from build123d import *

# Parameters (mm, degrees)
BOSS_EXTRUDE1_DEPTH     = 101
CUT_EXTRUDE1_START      = -32.5
SKETCH3_R               = 7.5
SKETCH3_R_2             = 5.975
CUT_EXTRUDE1_DEPTH      = 32.5
SKETCH4_R               = 7.5
SKETCH4_R_2             = 5.975
CUT_EXTRUDE2_DEPTH      = 32.5
CUT_EXTRUDE3_DEPTH      = 102.900993616
CUT_EXTRUDE3_DEPTH_BACK = 102.900993616
SKETCH5_W               = 8.2
SKETCH5_H               = 30.2
CUT_EXTRUDE4_DEPTH      = 103.382859894
CUT_EXTRUDE4_DEPTH_BACK = 103.382859894
HOLE1_D                 = 3.2
HOLE1_CSINK_D           = 6.3
HOLE1_CSINK_ANGLE       = 90


with BuildPart() as part:
    # Sketch1 → Boss-Extrude1 (new body)
    with BuildSketch(Plane.XY):
        with BuildLine():
            ThreePointArc((7.5, 0), (-1.941142838, 7.244443697), (-6.495190528, -3.75))
            Line((-6.495190528, -3.75), (6.495190528, -3.75))
            ThreePointArc((6.495190528, -3.75), (7.244443697, -1.941142838), (7.5, 0))
        make_face()
    extrude(amount=BOSS_EXTRUDE1_DEPTH)

    # Sketch3 → Cut-Extrude1 (cut)
    with BuildSketch(Plane.XY.offset(101).offset(CUT_EXTRUDE1_START)):
        Circle(SKETCH3_R)
        Circle(SKETCH3_R_2, mode=Mode.SUBTRACT)
    extrude(amount=CUT_EXTRUDE1_DEPTH, mode=Mode.SUBTRACT)

    # Sketch4 → Cut-Extrude2 (cut)
    with BuildSketch(Plane(origin=(0, 0, 0), x_dir=(-1, 0, 0), z_dir=(0, 0, -1))):
        Circle(SKETCH4_R)
        Circle(SKETCH4_R_2, mode=Mode.SUBTRACT)
    extrude(amount=-CUT_EXTRUDE2_DEPTH, mode=Mode.SUBTRACT)

    # Sketch5 → Cut-Extrude3 (cut, two sides: drawn at the far end of the back side and taken through both)
    with BuildSketch(Plane.XZ.offset(3.75).offset(-CUT_EXTRUDE3_DEPTH_BACK)):
        with Locations((0, 50.5)):
            Rectangle(SKETCH5_W, SKETCH5_H)
    extrude(amount=CUT_EXTRUDE3_DEPTH + CUT_EXTRUDE3_DEPTH_BACK, mode=Mode.SUBTRACT)

    # Sketch10 → Cut-Extrude4 (cut, two sides: drawn at the far end of the back side and taken through both)
    with BuildSketch(Plane.ZY.offset(7.5).offset(-CUT_EXTRUDE4_DEPTH_BACK)):
        with BuildLine():
            ThreePointArc((45.325, 2.112742786), (43.5, 3.937742786), (41.675, 2.112742786))
            Line((41.675, 2.112742786), (45.325, 2.112742786))
        make_face()
        with BuildLine():
            Line((45.325, 2.112742786), (41.675, 2.112742786))
            ThreePointArc((41.675, 2.112742786), (43.5, 0.287742786), (45.325, 2.112742786))
        make_face()
        with BuildLine():
            ThreePointArc((59.325, 2.112742786), (57.5, 3.937742786), (55.675, 2.112742786))
            Line((55.675, 2.112742786), (59.325, 2.112742786))
        make_face()
        with BuildLine():
            Line((59.325, 2.112742786), (55.675, 2.112742786))
            ThreePointArc((55.675, 2.112742786), (57.5, 0.287742786), (59.325, 2.112742786))
        make_face()
    extrude(amount=CUT_EXTRUDE4_DEPTH + CUT_EXTRUDE4_DEPTH_BACK, mode=Mode.SUBTRACT)

    # Hole1 (through all)
    with Locations(Plane(origin=(0, -3.75, 82.5), x_dir=(0, 0, -1), z_dir=(0, -1, 0))):
        with Locations((0, 0), (64, 0)):
            CounterSinkHole(HOLE1_D / 2, HOLE1_CSINK_D / 2, counter_sink_angle=HOLE1_CSINK_ANGLE)


solid = part.part
For this review, take the finished solid that the model builds, in its own axes (mm). A direction names the side the tool comes from. Round coordinates to 2 decimals unless told otherwise and drop trailing zeros. Loops run counter-clockwise (first coordinate to the right, second up) from the corner with the lowest first, then second, coordinate; pieces in that order, holes last. Notation, with made-up numbers: (0.5, 83.25) - (21.5, 83.25) arc R24 cw to (21.5, 99.25) - close; hole circle Ø10 at (-10, 63.25). An arc over 180 degrees is marked (long way). Put each result on its own line as item: value. Start each with the question number.
1. Consider section A-A on z = 82.5. State the section outline as (x, y) points (3 decimals).
2. For probe 1 along Z at (x, y) = (0, 3.5); probe 2 along X at (y, z) = (0.5, 35.5); probe 3 along Z at (x, y) = (-1.75, -1), list the stretches that pass through material, from the lowest coordinate up. Write a range as [from, to].
3. For faces 5 (the flat face through (4.1, 1, 50)), 6 (the cylindrical face through (5.8, 0.3, 57.7)), 7 (the cylindrical face through (-0.19, 5.97, 16.02)), list the 3-axis set-ups (+Z, -Z, +X, -X, +Y, -Y) from which the entire face can be reached by the end or side of a thin tool; tool diameter is ignored.
4. Consider section C-C on z = 57.5. State the section outline as (x, y) points.
5. Insertion check: P1, Ø1, axis at y = 5, z = 28, coming from the +X side; P2, Ø3.5, axis at x = 0, z = 82.5, coming from the +Y side (3 decimals); P3, Ø2, axis at y = 6.5, z = 61, coming from the -X side; P4, Ø3, axis at y = 2.11, z = 43.5, coming from the +X side. Each pin has a flat end and moves straight along its axis. Give the tip position at first contact, or say it passes through.
6. Consider section B-B on x = 0. State the section outline as (y, z) points (3 decimals).
7. Mouldability with a two-part tool opening along Z and no side actions: class faces 1 (the flat face through (0, 1, 101)), 2 (the flat face through (-4.4, -3.75, 49.8)), 3 (the cylindrical face through (5.8, 0.3, 43.7)), 4 (the flat face through (-4.1, 1, 50)) as +Z half, -Z half, draft (parallel to the pull), parting line (faces both ways), or undercut.
Result sheet:
1. outline: (-4.652, -3.75) - (-3.15, -3.75) - (-1.6, -2.2) - (-1.6, 5.757) arc R5.975 ccw to start; (1.6, -2.2) - (3.15, -3.75) - (4.652, -3.75) arc R5.975 ccw to (1.6, 5.757) - close
2. probe 1: [0, 16.9], [20.1, 35.4], [65.6, 80.9], [84.1, 101]
2. probe 2: [-7.48, -4.1], [4.1, 7.48]
2. probe 3: [0, 35.4], [65.6, 101]
3. face 5: +Y, -Y
3. face 6: +X, -X
3. face 7: -Z
4. outline: (-7.49, 0.29) arc R7.5 ccw to (-6.5, -3.75) - (-4.1, -3.75) - (-4.1, 0.29) - close; (-6.38, 3.94) - (-4.1, 3.94) - (-4.1, 6.28) arc R7.5 ccw to start; (4.1, -3.75) - (6.5, -3.75) arc R7.5 ccw to (7.49, 0.29) - (4.1, 0.29) - close; (4.1, 3.94) - (6.38, 3.94) arc R7.5 ccw to (4.1, 6.28) - close
5. P1: x = 3.93
5. P2: y = 5.975
5. P3: x = -5.1
5. P4: through
6. outline: (-3.75, 0) - (5.975, 0) - (5.975, 16.9) - (-2.2, 16.9) - (-3.75, 15.35) - close; (-3.75, 21.65) - (-2.2, 20.1) - (5.975, 20.1) - (5.975, 32.5) - (7.5, 32.5) - (7.5, 35.4) - (-3.75, 35.4) - close; (-3.75, 65.6) - (7.5, 65.6) - (7.5, 68.5) - (5.975, 68.5) - (5.975, 80.9) - (-2.2, 80.9) - (-3.75, 79.35) - close; (-3.75, 85.65) - (-2.2, 84.1) - (5.975, 84.1) - (5.975, 101) - (-3.75, 101) - close
7. face 1: +Z half
7. face 2: draft
7. face 3: undercut
7. face 4: undercut
